Here's how the part is built. I have some questions about the finished solid (model axes, mm). A direction names the side the tool comes from. Coordinates: 2 decimals unless noted, no trailing zeros. Write each loop counter-clockwise with the first axis right and the second up, starting at its lowest first coordinate (ties: lowest second). Pieces come first, ordered by that corner, then holes. Notation, with made-up numbers: (70.25, 73) -> (110.25, 73) arc R26 cw to (110.25, 94) -> close; hole circle Ø9 at (-13.75, 71.5). An arc over 180 degrees is marked (long way). Put each result on its own line as item: value.
```python
from build123d import *

# Parameters (mm, degrees)
EXTRUDE_1_DEPTH     = 7
SKETCH_1_2_W        = 20.1
SKETCH_1_2_H        = 49.6
EXTRUDE_2_DEPTH     = 2
SKETCH_2_W          = 3.45
SKETCH_2_H          = 1.5
EXTRUDE_3_DEPTH     = 3
SKETCH_3_R          = 0.75
SKETCH_3_W          = 13.2
SKETCH_3_H          = 1.7
SKETCH_3_W_2        = 12
CUT_EXTRUDE_1_DEPTH = 2
FILLET_1_R          = 1.5
FILLET_2_R          = 1.5


with BuildPart() as part:
    # Sketch 1 → Extrude 1 (new body)
    with BuildSketch(Plane.XY):
        with BuildLine():
            ThreePointArc((1.7, -27.866190379), (0.542893219, -27.730776406), (0, -26.7))
            Line((0, -26.7), (0, -53))
            Line((0, -53), (23.5, -53))
            Line((23.5, -53), (23.5, -26.7))
            ThreePointArc((23.5, -26.7), (22.957106781, -27.730776406), (21.8, -27.866190379))
            Line((21.8, -27.866190379), (21.8, -51.3))
            Line((21.8, -51.3), (1.7, -51.3))
            Line((1.7, -51.3), (1.7, -27.866190379))
        make_face()
        with BuildLine():
            ThreePointArc((1.7, -25.533809621), (0.542893219, -25.669223594), (0, -26.7))
            ThreePointArc((0, -26.7), (0.542893219, -27.730776406), (1.7, -27.866190379))
            Line((1.7, -27.866190379), (1.7, -25.533809621))
        make_face()
        with BuildLine():
            ThreePointArc((2.5, -26.7), (2.280776406, -25.992893219), (1.7, -25.533809621))
            Line((1.7, -25.533809621), (1.7, -27.866190379))
            ThreePointArc((1.7, -27.866190379), (2.280776406, -27.407106781), (2.5, -26.7))
        make_face()
        with BuildLine():
            Line((23.5, 0), (0, 0))
            Line((0, 0), (0, -26.7))
            ThreePointArc((0, -26.7), (0.542893219, -25.669223594), (1.7, -25.533809621))
            Line((1.7, -25.533809621), (1.7, -1.7))
            Line((1.7, -1.7), (21.8, -1.7))
            Line((21.8, -1.7), (21.8, -25.533809621))
            ThreePointArc((21.8, -25.533809621), (22.957106781, -25.669223594), (23.5, -26.7))
            Line((23.5, -26.7), (23.5, 0))
        make_face()
        with BuildLine():
            ThreePointArc((21.8, -27.866190379), (22.957106781, -27.730776406), (23.5, -26.7))
            ThreePointArc((23.5, -26.7), (22.957106781, -25.669223594), (21.8, -25.533809621))
            Line((21.8, -25.533809621), (21.8, -27.866190379))
        make_face()
        with BuildLine():
            Line((21.8, -27.866190379), (21.8, -25.533809621))
            ThreePointArc((21.8, -25.533809621), (21, -26.7), (21.8, -27.866190379))
        make_face()
    extrude(amount=EXTRUDE_1_DEPTH)

    # Sketch 1_2 → Extrude 2 (add)
    with BuildSketch(Plane.XY):
        with Locations((11.75, -26.5)):
            Rectangle(SKETCH_1_2_W, SKETCH_1_2_H)
    extrude(amount=EXTRUDE_2_DEPTH)

    # Sketch 2 → Extrude 3 (add)
    with BuildSketch(Plane.XY.offset(2)):
        with Locations((3.425, -43.05)):
            Rectangle(SKETCH_2_W, SKETCH_2_H)
        with Locations((20.075, -43.05)):
            Rectangle(SKETCH_2_W, SKETCH_2_H)
        with Locations((3.425, -9.95)):
            Rectangle(SKETCH_2_W, SKETCH_2_H)
        with Locations((20.075, -9.95)):
            Rectangle(SKETCH_2_W, SKETCH_2_H)
    extrude(amount=EXTRUDE_3_DEPTH)

    # Sketch 3 → Cut-Extrude 1 (cut)
    with BuildSketch(Plane.XY.offset(7)):
        with Locations((22.25, -26.7)):
            Circle(SKETCH_3_R)
        with Locations((1.25, -26.7)):
            Circle(SKETCH_3_R)
        with Locations((11.75, -52.15)):
            Rectangle(SKETCH_3_W, SKETCH_3_H)
        with Locations((11.75, -0.85)):
            Rectangle(SKETCH_3_W_2, SKETCH_3_H)
    extrude(amount=-CUT_EXTRUDE_1_DEPTH, mode=Mode.SUBTRACT)

    # Fillet 1
    fillet_1_edges = [part.edges().sort_by_distance(p)[0] for p in [
        (23.5, -53, 3.5),
        (0, -53, 3.5),
        (0, 0, 3.5),
        (23.5, 0, 3.5),
    ]]
    fillet(fillet_1_edges, radius=FILLET_1_R)

    # Fillet 2
    fillet_2_edges = [part.edges().sort_by_distance(p)[0] for p in [
        (0, -26.5, 0),
        (11.75, -53, 0),
        (11.75, 0, 0),
        (23.5, -26.5, 0),
        (0.439339828, -52.560660172, 0),
        (23.060660172, -52.560660172, 0),
        (23.060660172, -0.439339828, 0),
        (0.439339828, -0.439339828, 0),
    ]]
    fillet(fillet_2_edges, radius=FILLET_2_R)


solid = part.part
```
Item 1: Imagine slicing it at B-B on x = 4. Write out the boundary of the cut face in (y, z).
Output:
outline: (-53, 1.5) arc R1.5 ccw to (-51.5, 0) -> (-1.5, 0) arc R1.5 ccw to (0, 1.5) -> (0, 7) -> (-1.7, 7) -> (-1.7, 2) -> (-9.2, 2) -> (-9.2, 5) -> (-10.7, 5) -> (-10.7, 2) -> (-42.3, 2) -> (-42.3, 5) -> (-43.8, 5) -> (-43.8, 2) -> (-51.3, 2) -> (-51.3, 7) -> (-53, 7) -> close
Item 2: Which directions (+Z, -Z, +X, -X, +Y, -Y) give clear straight access to the entire face, cutting with the end or side of a thin tool? Please do faces 1 (the cylindrical face through (23.07, -0.45, 4.29)), 2 (the flat face through (20, -10.7, 3)), 3 (the flat face through (18.35, -52, 6)).
Output:
face 1: +Z, -Z, +X, +Y
face 2: +Z
face 3: +Z, -Y
Item 3: Imagine slicing it at D-D on x = 8.25. Write out the boundary of the cut face in (y, z).
Output:
outline: (-53, 1.5) arc R1.5 ccw to (-51.5, 0) -> (-1.5, 0) arc R1.5 ccw to (0, 1.5) -> (0, 5) -> (-1.7, 5) -> (-1.7, 2) -> (-51.3, 2) -> (-51.3, 5) -> (-53, 5) -> close
Item 4: Imagine slicing it at C-C on y = -3. Write out the boundary of the cut face in (x, z), then the cut area to 3 significant figures.
Output:
outline: (0, 1.5) arc R1.5 ccw to (1.5, 0) -> (22, 0) arc R1.5 ccw to (23.5, 1.5) -> (23.5, 7) -> (21.8, 7) -> (21.8, 2) -> (1.7, 2) -> (1.7, 7) -> (0, 7) -> close
area: 63.0 mm²
Item 5: For P1, Ø1.4, axis at y = -0.5, z = 6, coming from the -X side; P2, Ø10, axis at x = 12, y = -26, coming from the +Z side, each with a flat end and sliding along its axis, tell me the tip position at first contact or that it passes through.
Output:
P1: stops at x = 0.03
P2: stops at z = 2
Item 6: If we mould it in two halves opening along Y, with no side actions, what happens to faces 4 (the cylindrical face through (23.07, -52.55, 4.29)), 5 (the cylindrical face through (0.45, -0.43, 4.29)), 6 (the flat face through (12, -26, 0)), 7 (the flat face through (1.7, -14, 4))? For each: released by +Y, released by -Y, zero draft, split by the parting line, or undercut.
Output:
face 4: released by -Y
face 5: released by +Y
face 6: zero draft
face 7: undercut
Item 7: Imagine slicing it at A-A on z = 6. Write out the boundary of the cut face in (x, y), then the cut area to 3 significant figures.
Output:
outline: (0, -51.5) arc R1.5 ccw to (1.5, -53) -> (5.15, -53) -> (5.15, -51.3) -> (1.7, -51.3) -> (1.7, -27.87) arc R1.25 ccw to (1.7, -25.53) -> (1.7, -1.7) -> (5.75, -1.7) -> (5.75, 0) -> (1.5, 0) arc R1.5 ccw to (0, -1.5) -> close; (17.75, -1.7) -> (21.8, -1.7) -> (21.8, -25.53) arc R1.25 ccw to (21.8, -27.87) -> (21.8, -51.3) -> (18.35, -51.3) -> (18.35, -53) -> (22, -53) arc R1.5 ccw to (23.5, -51.5) -> (23.5, -1.5) arc R1.5 ccw to (22, 0) -> (17.75, 0) -> close; hole circle Ø1.5 at (1.25, -26.7); hole circle Ø1.5 at (22.25, -26.7)
area: 203 mm²
Item 8: Please list where these lines run through material, in increasing order: line 1 along Y through (x, z) = (2.75, 6); line 2 along X through (y, z) = (-49.5, 5.75); line 3 along Y through (x, z) = (1.75, 4.5). Write a range as from..to.
Output:
line 1: y = -53..-51.3, -1.7..0
line 2: x = 0..1.7, 21.8..23.5
line 3: y = -53..-51.3, -43.8..-42.3, -27.85..-25.55, -10.7..-9.2, -1.7..0
